For this review, take the finished solid that the model builds, in its own axes (mm). Face numbers are marked on the shaded views. A direction names the side the tool comes from. Give positions to 0.01 mm unless a question says otherwise; leave off trailing zeros. Order: outer loops, then holes, each group sorted by start corner. A loop starts at its lowest first (then second) coordinate and runs counter-clockwise, first axis right, second up.
Item 1: Consider section C-C (z = -6). Give the boundary of the cut face in (x, y).
Item 2: Consider section A-A (y = 34). Give the boundary of the cut face in (x, z), plus the area to 3 significant figures.
Item 3: For P1, Ø20, axis at x = -175.55, z = -42.85, coming from the +Y side; P2, Ø8, axis at x = -136.4, y = 25.9, coming from the -Z side; P3, Ø21, axis at x = -156, z = -75.5, coming from the +Y side, all flat-tipped, find the tip position at first contact; note any pin that passes through.
Item 4: Machinability: for the marked faces 1, 2 and 3, which of the approach directions +Z, -Z, +X, -X, +Y, -Y give a long, thin tool a straight path to every point of the face, cutting with its end or side? Answer none if there is none.
Item 5: The part is to be moulded in two halves that separate along X. For the marked faces 4, 5 and 6, say which applies: released by +X, released by -X, zero draft, split by the parting line, or undercut.
Item 6: For probe 1 along Y at (x, z) = (1.5, -43.7); probe 2 along X at (y, z) = (2.9, -44); probe 3 along Z at (x, y) = (-39.5, 13.5), list the stretches that pass through material, from the lowest coordinate up.
Item 7: Consider section B-B (x = -54.5). Give the boundary of the cut face in (y, z).
Item 8: Consider section D-D (y = 12). Give the boundary of the cut face in (x, z).
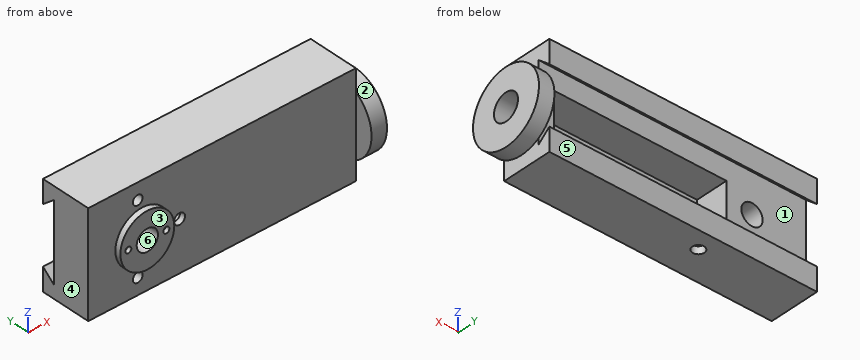
Autodesk Inventor part; units mm, degrees
ref_plane "YZ Plane" through (0, 0, 0) normal (1, 0, 0) x (0, 1, 0)
ref_plane "XZ Plane" through (0, 0, 0) normal (0, 1, 0) x (-1, 0, 0)
ref_plane "XY Plane" through (0, 0, 0) normal (0, 0, 1) x (1, 0, 0)
sketch "Sketch1" plane through (0, 0, 0) normal (1, 0, 0) x (0, 1, 0)
  line L0 (0, 0) -> (0, -85)
  line L1 (0, -85) -> (41.4, -85)
  line L2 (41.4, -85) -> (41.4, 0)
  line L3 (41.4, 0) -> (0, 0)
  dimension "d0" = 85
  dimension "d1" = 41.4
extrude "Extrusion1" add sketch "Sketch1" against normal blind 220
sketch "Sketch2" plane through (0, 0, 0) normal (1, 0, 0) x (0, 0, -1)
  line L0 (0, 41.4) -> (19, 41.4)
  line L1 (10.609, 31.4) -> (19, 41.4)
  line L2 (10.609, 31.4) -> (74.391, 31.4)
  line L3 (85, 41.4) -> (66, 41.4)
  line L4 (66, 41.4) -> (74.391, 31.4)
  line L5 (19, 41.4) -> (66, 41.4)
  line L6 (0, 41.4) -> (85, 41.4)
  line L7 (42.5, 41.4) -> (42.5, 31.4) construction
  dimension "d4" = 19
  dimension "d8" = 19
  dimension "d61" = 50
  dimension "d63" = 50
  dimension "d64" = 10
extrude "Extrusion2" cut sketch "Sketch2" against normal blind 301.25
sketch "Sketch3" plane through (0, 31.4, -10.609) normal (0, 1, 0) x (1, 0, 0)
  line L0 (0, -10.609) -> (0, 74.391)
  line L1 (-12.6, 32) -> (-12.6, 47.1)
  line L2 (-12.6, 32) -> (-12.6, 16.9)
  line L3 (-12.6, 16.9) -> (-154.5, 16.9)
  line L4 (-154.5, 16.9) -> (-154.5, 47.1)
  line L5 (-154.5, 47.1) -> (-12.6, 47.1)
  dimension "d12" = 15.1
  dimension "d13" = 15.1
  dimension "d14" = 141.9
extrude "Extrusion3" cut sketch "Sketch3" against normal blind 26.9
sketch "Sketch4" plane through (0, 31.4, -10.609) normal (0, 1, 0) x (1, 0, 0)
  point P0 (0, -10.609)
sketch "Sketch5" plane through (0, 0, 0) normal (1, 0, 0) x (0, 0, -1)
  line L0 (0, 41.4) -> (0, 0)
  line L1 (0, 0) -> (28.6, 0)
  line L2 (85, 0) -> (0, 0)
  line L3 (28.6, 0) -> (58.8, 0)
  line L4 (85, 41.4) -> (85, 0)
  line L5 (58.8, 0) -> (85, 0)
  line L6 (28.6, 0) -> (43.7, 0)
  line L7 (43.7, 0) -> (43.7, 31.4)
  line L8 (27.509, 31.4) -> (57.709, 31.4)
  line L9 (43.7, 31.4) -> (43.7, 26.8)
  line L10 (43.7, 26.8) -> (43.7, 14.6)
  line L11 (43.7, 26.8) -> (43.7, 15.8)
  circle A0 centre (43.7, 15.8) radius 11
  dimension "d17" = 28.6
  dimension "d18" = 30.2
  dimension "d19" = 4.6
  dimension "d21" = 11
extrude "Extrusion4" cut sketch "Sketch5" against normal blind 91.9
sketch "Sketch6" plane through (0, 0, 0) normal (1, 0, 0) x (0, 0, -1)
  point P0 (0, 0)
sketch "Sketch7" plane through (0, 0, 0) normal (1, 0, 0) x (0, 0, -1)
  circle A0 centre (43.7, 15.8) radius 11
  circle A1 centre (43.7, 15.8) radius 30.2
  point P0 (0, 0)
  dimension "d24" = 60.4
extrude "Extrusion5" add sketch "Sketch7" along normal blind 12.7
sketch "Sketch8" plane through (0, 0, -85) normal (0, 0, -1) x (-1, 0, 0)
  line L0 (220, 31.4) -> (220, 41.4)
  line L1 (220, 41.4) -> (220, 30.8)
  line L2 (220, 41.4) -> (220, 0)
  line L3 (220, 30.8) -> (136.4, 30.8)
  line L4 (154.5, 31.4) -> (12.6, 31.4)
  line L5 (136.4, 30.8) -> (136.4, 25.9)
  line L6 (0, 0) -> (220, 0)
  circle A0 centre (136.4, 25.9) radius 4.9
  dimension "d27" = 10.6
  dimension "d28" = 83.6
  dimension "d29" = 90
  dimension "d30" = 4.9
extrude "Extrusion6" cut sketch "Sketch8" against normal blind 6
sketch "Sketch9" plane through (-220, 0, 0) normal (0, -1, 0) x (1, 0, 0)
  line L0 (0, -85) -> (0, 0)
  line L1 (0, -85) -> (0, -63)
  line L2 (0, -63) -> (22.3, -63)
  line L3 (0, 0) -> (0, -22.7)
  line L4 (0, -22.7) -> (22.3, -22.7)
  line L5 (22.3, -22.7) -> (22.3, -63)
  line L6 (22.3, -42.85) -> (44.45, -42.85)
  line L7 (65.5, -27.509) -> (65.5, -57.709)
  line L8 (22.3, -42.85) -> (44.45, -42.85) construction
  circle A0 centre (44.45, -42.85) radius 22.15
  point P0 (220, 0)
  dimension "d33" = 22
  dimension "d34" = 22.3
  dimension "d35" = 22.7
  dimension "d36" = 22.15
  dimension "d37" = 0
extrude "Extrusion7" add sketch "Sketch9" along normal blind 4.6 contours A0 L7 | A0 L7
sketch "Sketch10" plane through (-175.55, -4.6, -42.85) normal (0, -1, 0) x (1, 0, 0)
  circle A0 centre (0, 0) radius 8.75
  point P0 (175.55, 42.85)
  dimension "d40" = 17.5
extrude "Extrusion8" cut sketch "Sketch10" against normal blind 310.85
sketch "Sketch11" plane through (-175.55, -4.6, -42.85) normal (0, -1, 0) x (1, 0, 0)
  circle A0 centre (0, 0) radius 8.75
  line L0 (-8.75, 0) -> (-13.15, 0)
  line L1 (-13.15, 0) -> (-18.15, 0)
  circle A1 centre (-15.65, 0) radius 2.5
  line L2 (8.75, 0) -> (13.15, 0)
  line L3 (13.15, 0) -> (15.65, 0)
  circle A2 centre (15.65, 0) radius 2.5
  point P0 (175.55, 42.85)
  dimension "d43" = 4.4
  dimension "d44" = 5
  dimension "d45" = 4.4
  dimension "d46" = 2.5
extrude "Extrusion9" cut sketch "Sketch11" against normal blind 3.5 contours A1 L1 | L1 A1 | A2
sketch "Sketch12" plane through (-220, 0, 0) normal (0, -1, 0) x (1, 0, 0)
  line L0 (0, 0) -> (40.7, 0)
  line L1 (220, 0) -> (0, 0)
  line L2 (40.7, 0) -> (40.7, -9.4)
  line L3 (40.7, -9.4) -> (40.7, -13.4)
  circle A0 centre (40.7, -13.4) radius 4
  line L4 (220, -85) -> (0, -85)
  line L5 (0, -85) -> (40.7, -85)
  line L6 (40.7, -85) -> (40.7, -75.6)
  line L7 (40.7, -75.6) -> (40.7, -71.6)
  circle A1 centre (40.7, -71.6) radius 4
  line L8 (0, 0) -> (70.6, 0)
  line L9 (70.6, 0) -> (70.6, -39.5)
  line L10 (70.6, -39.5) -> (70.6, -44)
  line L11 (70.6, -39.5) -> (75.1, -39.5)
  line L12 (75.1, -39.5) -> (75.1, -44)
  circle A2 centre (75.1, -44) radius 4.5
  dimension "d49" = 40.7
  dimension "d50" = 9.4
  dimension "d51" = 4
  dimension "d52" = 40.7
  dimension "d53" = 9.4
  dimension "d54" = 4
  dimension "d55" = 70.6
  dimension "d56" = 39.5
  dimension "d57" = 4.5
  dimension "d58" = 4.5
extrude "Extrusion10" cut sketch "Sketch12" against normal blind 7 contours A0 | A2 | A1
properties part number "Bottom Tool Bit" material "Steel, Cast"
Resolved:
1. outline: (-220, 0) - (0, 0) - (0, 41.4) - (-220, 41.4) - close
2. outline: (-220, -85) - (0, -85) - (0, -72.21) - (-220, -72.21) - close; (-220, -12.79) - (0, -12.79) - (0, 0) - (-220, 0) - close; (0, -67.8) - (12.7, -67.8) - (12.7, -19.6) - (0, -19.6) - close
2. area: 6,240 mm2
3. P1: stops at y = 31.4
3. P2: stops at z = -79
3. P3: stops at y = 41.4
4. face 1: -X
4. face 2: +X
4. face 3: +Z, -Z, -X, -Y
5. face 4: released by -X
5. face 5: zero draft
5. face 6: undercut
6. probe 1: y = -14.4 to 4.8, 26.8 to 46
6. probe 2: x = -220 to -184.22, -166.88 to -149.4, -140.4 to 12.7
6. probe 3: z = -85 to -57.71, -27.51 to 0
7. outline: (0, -85) - (41.4, -85) - (41.4, -66) - (31.4, -74.39) - (31.4, -57.71) - (4.5, -57.71) - (4.5, -27.51) - (31.4, -27.51) - (31.4, -10.61) - (41.4, -19) - (41.4, 0) - (0, 0) - close
8. outline: (-220, -85) - (0, -85) - (0, -73.66) - (12.7, -73.66) - (12.7, -54.02) - (-12.6, -54.02) - (-12.6, -57.71) - (-154.5, -57.71) - (-154.5, -27.51) - (-12.6, -27.51) - (-12.6, -33.38) - (12.7, -33.38) - (12.7, -13.74) - (0, -13.74) - (0, 0) - (-220, 0) - close; hole circle Ø17.5 at (-175.55, -42.85)
